Part print with two shaded views. Sizes in mm from the minimum x, y, z corner. A direction names the side the tool comes from. Give positions to 0.01 mm unless a question says otherwise; leave off trailing zeros. Write each loop counter-clockwise with the first axis right and the second up, starting at its lowest first coordinate (ties: lowest second). Pieces come first, ordered by that corner, then holes. Notation, with made-up numbers: (66, 80) -> (116, 80) arc R21 cw to (116, 105) -> close; hole circle Ø9 at (4.25, -24.5). An arc over 180 degrees is marked (long way). Use one line per item in the form item = value. Start each with the question number.
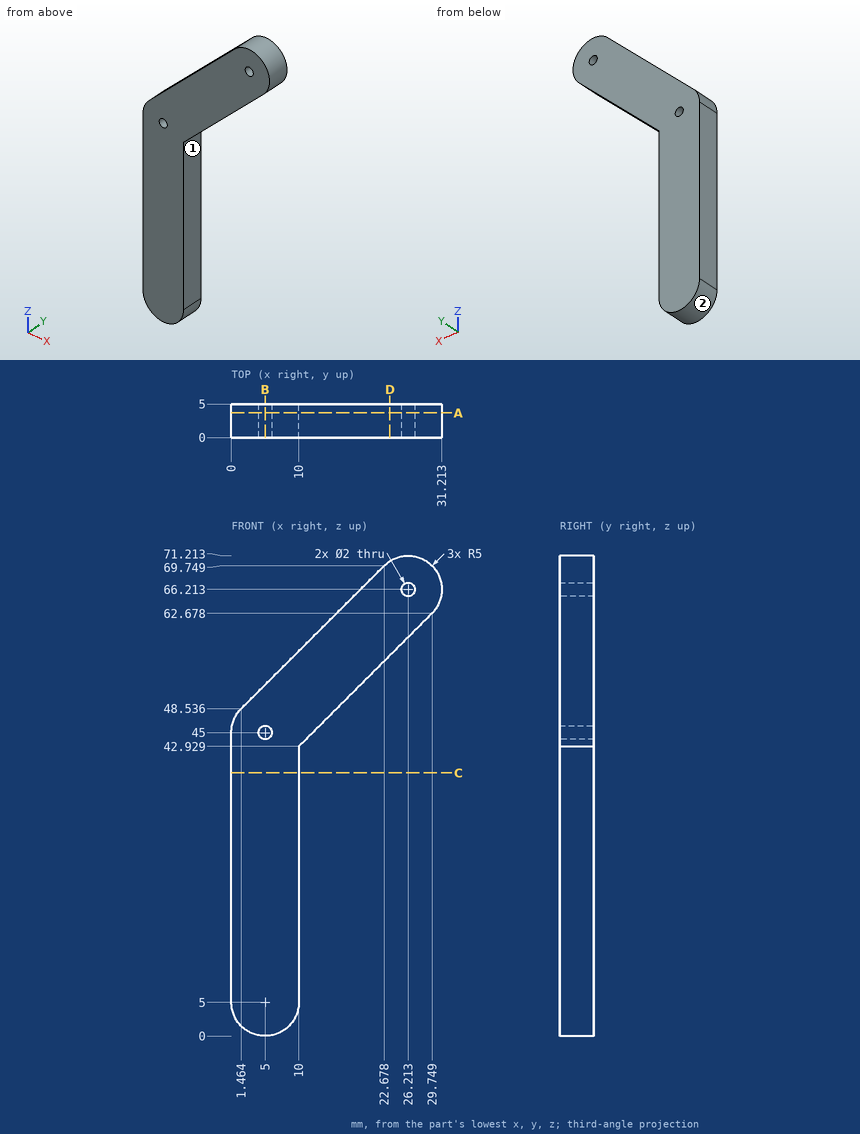
1) Cut at C-C (z = 39). Give the cut face in (x, y), and give its area (3 significant figures).
2) Cut at B-B (x = 5). Give the cut face in (y, z), and give its area (3 significant figures).
3) Cut at A-A (y = 3.7). Give the cut face in (x, z) (1 decimal).
4) Wall check: line 1 along X through (y, z) = (2.5, 29); line 2 along X through (y, z) = (1.35, 45); line 3 along Z through (x, y) = (20, 4.35). Give the ranges that are in metal, low to high. Write a range as from..to.
5) Pin check, flat tips, straight feed: pin 1 (1 mm diameter, centred on y = 1, z = 60, fed in from -X); pin 2 (2 mm diameter, centred on y = 1, z = 47, fed in from +X). Stop position of each tip, or through.
6) Cut at D-D (x = 23.5). Give the cut face in (y, z).
7) 3-axis set-ups, long thin cutter, end or side, ignore diameter. For the marked faces 1 and 2: which of +Z, -Z, +X, -X, +Y, -Y reach the whole face in a straight line?
Final values:
q1.outline = (0, 0) -> (10, 0) -> (10, 5) -> (0, 5) -> close
q1.area = 50.0 mm^2
q2.outline = (0, 0) -> (5, 0) -> (5, 44) -> (0, 44) -> close; (0, 46) -> (5, 46) -> (5, 52.07) -> (0, 52.07) -> close
q2.area = 250 mm^2
q3.outline = (0, 5) arc R5 ccw to (10, 5) -> (10, 42.9) -> (29.7, 62.7) arc R5 ccw to (22.7, 69.7) -> (1.5, 48.5) arc R5 ccw to (0, 45) -> close; hole circle Ø2 at (5, 45); hole circle Ø2 at (26.2, 66.2)
q4.line_1 = 0..10
q4.line_2 = 0..4, 6..12.07
q4.line_3 = 52.93..67.07
q5.pin_1 = 12.43
q5.pin_2 = 15.07
q6.outline = (0, 56.43) -> (5, 56.43) -> (5, 70.41) -> (0, 70.41) -> close
q7.face_1 = -Z, +X, +Y, -Y
q7.face_2 = -Z, +Y, -Y
